Autodesk Inventor part; units mm, degrees
ref_plane "Work Plane1" through (0, 0, 40) normal (0, 0, 1) x (1, 0, 0)
ref_plane "YZ Plane" through (0, 0, 0) normal (1, 0, 0) x (0, 1, 0)
ref_plane "XZ Plane" through (0, 0, 0) normal (0, 1, 0) x (-1, 0, 0)
sketch "Sketch1" plane through (0, 0, 0) normal (0, 0, 1) x (1, 0, 0)
  line L0 (0, 0) -> (40, 0)
  line L1 (40, 0) -> (40, 50)
  line L2 (40, 50) -> (0, 50)
  line L3 (0, 50) -> (0, 0)
  dimension "d0" = 40
  dimension "d1" = 50
extrude "Extrusion1" add sketch "Sketch1" along normal blind 30
sketch "Sketch2" plane through (0, 0, 30) normal (0, 0, 1) x (1, 0, 0)
  circle A0 centre (20, 25) radius 10
ref_plane "Work Plane1" through (0, 0, 40) normal (0, 0, 1) x (1, 0, 0)
sketch "Sketch3" plane through (0, 0, 40) normal (0, 0, 1) x (1, 0, 0)
  circle A0 centre (20, 25) radius 15
  point P0 (0, 0)
  dimension "d6" = 30
loft "Loft1" add profiles "Sketch3", "Sketch2"
properties part number "Camera"
Geometry check sheet. Reference: the model listing, model coordinates, mm. A direction names the side the tool comes from. Coordinates: 2 decimals unless noted, no trailing zeros. Write each loop counter-clockwise with the first axis right and the second up, starting at its lowest first coordinate (ties: lowest second). Pieces come first, ordered by that corner, then holes. Notation, with made-up numbers: M 51,-17 L 105,-17 A21 cw 105,15 Z; hole C 52,-22.75 d8. An arc over 180 degrees is marked long. Answer as a JSON object with one key per item and string values.
1. Section check A-A, the plane x = 20. Enter the section's corners in (y, z), plus the area to 3 significant figures.
Answers below:
{"outline": "M 0,0 L 50,0 L 50,30 L 35,30 L 40,40 L 10,40 L 15,30 L 0,30 Z", "area": "1,750 mm²"}
2. Section check B-B, the plane y = 45. Enter the section's corners in (x, z), plus the area to 3 significant figures.
Answers below:
{"outline": "M 0,0 L 40,0 L 40,30 L 0,30 Z", "area": "1,200 mm²"}
3. Tool access check on faces 1 (the conical face through (24.76, 15.85, 30.63)), 2 (the flat face through (40, 25, 15)). Record the directions out of +Z, -Z, +X, -X, +Y, -Y that give a thin tool (end or side, any length) a straight path to the whole face; none if there is none.
Answers below:
{"face 1": "none", "face 2": "+Z, -Z, +X, +Y, -Y"}
4. Go/stop test with flat-tipped pins: pin 1 Ø4 at (y, z) = (10, 20.5) entering from -X; pin 2 Ø6 at (x, y) = (31.5, 44.5) entering from +Z. Record where each tip stops, or that it passes through.
Answers below:
{"pin 1": "stops at x = 0", "pin 2": "stops at z = 30"}
5. Scan lines: L1, parallel to Z at x = 36, y = 28.5; L2, parallel to X at y = 29, z = 31; L3, parallel to Z at x = 12, y = 34. Record each from-to range of solid material in increasing order.
Answers below:
{"L1": "z = 0 to 30", "L2": "x = 10.29 to 29.71", "L3": "z = 0 to 30, 34.08 to 40"}
